from build123d import *

# Parameters (mm, degrees)
SKETCH027_W     = 30
SKETCH027_H     = 30
PAD013_DEPTH    = 4.7
POCKET011_DEPTH = 3.501
PAD014_DEPTH    = 1.2
SKETCH031_R     = 2.5
POCKET012_DEPTH = 91.570364


with BuildPart() as part:
    # Sketch027 → Pad013 (new body)
    with BuildSketch(Plane.XY):
        Rectangle(SKETCH027_W, SKETCH027_H)
    extrude(amount=PAD013_DEPTH)

    # Sketch028 → Pocket011 (cut, through all)
    with BuildSketch(Plane.XY.offset(1.2)):
        with BuildLine():
            Line((-6, 1.75), (-15, 1.75))
            Line((-15, 1.75), (-15, -1.75))
            Line((-6, -1.75), (-15, -1.75))
            ThreePointArc((-6, -1.75), (-0.702489, 0.337963), (1.745834, 5.47887))
            ThreePointArc((5.47887, 1.745834), (7.712375, 7.712375), (1.745834, 5.47887))
            ThreePointArc((5.47887, 1.745834), (0.337963, -0.702489), (-1.75, -6))
            Line((-1.75, -6), (-1.75, -15))
            Line((1.75, -15), (-1.75, -15))
            Line((1.75, -6), (1.75, -15))
            ThreePointArc((5.72024, -1.745834), (2.896751, -3.090501), (1.75, -6))
            ThreePointArc((5.72024, -1.745834), (10.187248, 10.187248), (-1.745834, 5.72024))
            ThreePointArc((-6, 1.75), (-3.090501, 2.896751), (-1.745834, 5.72024))
        make_face()
    extrude(amount=POCKET011_DEPTH, mode=Mode.SUBTRACT)

    # Sketch029 → Pad014 (join)
    with BuildSketch(Plane.XY.offset(4.7)):
        Polygon((15, -15), (15, 15), (-15, 15), (-15, 1.75), (-13.4, 1.75), (-13.4, 13.4), (13.4, 13.4), (13.4, -13.4), (1.75, -13.4), (1.75, -15), align=None)
        Polygon((-1.75, -15), (-15, -15), (-15, -1.75), (-13.4, -1.75), (-13.4, -13.4), (-1.75, -13.4), align=None)
    extrude(amount=PAD014_DEPTH)

    # Sketch031 → Pocket012 (cut, through all)
    with BuildSketch(Plane.XY):
        with Locations((-8, -8)):
            Circle(SKETCH031_R)
    pocket012 = extrude(amount=POCKET012_DEPTH, mode=Mode.SUBTRACT)

    # Mirrored004: Pocket012 across Sketch031 V_Axis
    add(pocket012.mirror(Plane(origin=(0, 0, 0), x_dir=(0, 0, 1), z_dir=(1, 0, 0))), mode=Mode.SUBTRACT)

    # Mirrored005: Pocket012 across Sketch031 H_Axis
    add(pocket012.mirror(Plane.ZX), mode=Mode.SUBTRACT)


solid = part.part
For this review, take the finished solid that the model builds, in its own axes (mm). A direction names the side the tool comes from. Give positions to 0.01 mm unless a question says otherwise; leave off trailing zeros. Order: outer loops, then holes, each group sorted by start corner. A loop starts at its lowest first (then second) coordinate and runs counter-clockwise, first axis right, second up. Notation, with made-up numbers: M 71.25,-36 L 92.25,-36 A5 cw 92.25,-28 Z; hole C 52.25,31.25 d4. An arc over 180 degrees is marked long. Answer in a Markdown table with one row per item. Add a question column.
(1) Consider section D-D on y = 9.5. State the section outline as (x, z) points, and give its area (3 significant figures).
(2) For faces 1 (the face through (1.75, -10, 3)), 2 (the face through (-13.4, 7, 5)), 3 (the face through (-8.54, 10.44, 2.32)), list the 3-axis set-ups (+Z, -Z, +X, -X, +Y, -Y) from which the entire face can be reached by the end or side of a thin tool; tool diameter is ignored.
(3) Consider section A-A on x = -8. State the section outline as (y, z) points.
(4) For pin 1 (2 mm diameter, centred on x = 2, y = -1.5, fed in from -Z); pin 2 (1.5 mm diameter, centred on x = 0.5, z = 4, fed in from -Y); pin 3 (6.5 mm diameter, centred on x = 8, y = -8, fed in from +Z); pin 4 (1.3 mm diameter, centred on x = 1, z = 5, fed in from -Y), all flat-tipped, find the tip position at first contact; note any pin that passes through.
(5) Wall thickness on probe 1 along Y at (x, z) = (-8, 1.15); probe 2 along Y at (x, z) = (-8, 1.95); probe 3 along Y at (x, z) = (-7, 5.55): over which ranges is each line inside the solid? List them lowest first. Write a range as [from, to].
(6) Consider section B-B on z = 3.5. State the section outline as (x, y) points.
(7) Mouldability with a two-part tool opening along X and no side actions: class faces 4 (the face through (-10, -1.75, 3)), 5 (the face through (0.394, -0.643, 2.926)) as +X half, -X half, draft (parallel to the pull), parting line (faces both ways), or undercut.
Evaluation:
| question | item | result |
|---|---|---|
| 1 | outline | M -15,0 L -10,0 L -10,4.7 L -13.4,4.7 L -13.4,5.9 L -15,5.9 Z; M -6,0 L 15,0 L 15,5.9 L 13.4,5.9 L 13.4,4.7 L 10.79,4.7 L 10.79,1.2 L -0.32,1.2 L -0.32,4.7 L -6,4.7 Z |
| 1 | area | 87.2 mm^2 |
| 2 | face 1 | +Z, -Y |
| 2 | face 2 | +Z |
| 2 | face 3 | +Z, -Z |
| 3 | outline | M -15,0 L -10.5,0 L -10.5,4.7 L -13.4,4.7 L -13.4,5.9 L -15,5.9 Z; M -5.5,0 L 5.5,0 L 5.5,4.7 L 1.75,4.7 L 1.75,1.2 L -1.75,1.2 L -1.75,4.7 L -5.5,4.7 Z; M 10.5,0 L 15,0 L 15,5.9 L 13.4,5.9 L 13.4,4.7 L 10.5,4.7 Z |
| 4 | pin 1 | stops at z = 0 |
| 4 | pin 2 | stops at y = -1.41 |
| 4 | pin 3 | stops at z = 4.7 |
| 4 | pin 4 | stops at y = -0.61 |
| 5 | probe 1 | y = [-15, -10.5], [-5.5, 5.5], [10.5, 15] |
| 5 | probe 2 | y = [-15, -10.5], [-5.5, -1.75], [1.75, 5.5], [10.5, 15] |
| 5 | probe 3 | y = [-15, -13.4], [13.4, 15] |
| 6 | outline | M -15,-15 L -1.75,-15 L -1.75,-6 A7.76 cw 5.48,1.75 A3.5 ccw long 1.75,5.48 A7.76 cw -6,-1.75 L -15,-1.75 Z; M -15,1.75 L -6,1.75 A4.26 ccw -1.75,5.72 A7 cw long 5.72,-1.75 A4.26 ccw 1.75,-6 L 1.75,-15 L 15,-15 L 15,15 L -15,15 Z; hole C -8,-8 d5; hole C -8,8 d5; hole C 8,-8 d5 |
| 7 | face 4 | draft |
| 7 | face 5 | undercut |
